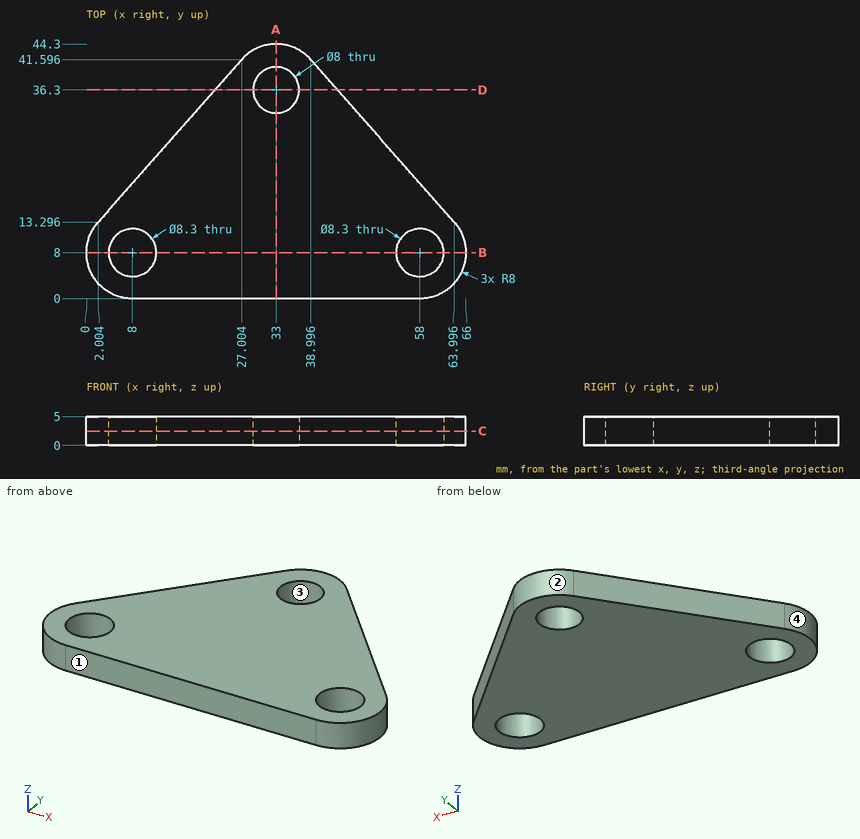
Check sheet for the drawn part. Datum: minimum x, y, z corner. Units: mm. Give positions to 0.01 mm unless a question says otherwise; leave off trailing zeros. Write each loop counter-clockwise with the first axis right and the second up, starting at its lowest first coordinate (ties: lowest second). Pieces come first, ordered by that corner, then holes. Notation, with made-up numbers: (26, 22.25) -> (69, 22.25) arc R7 cw to (69, 32.25) -> close; hole circle Ø11 at (9, 53.5). An arc over 180 degrees is marked (long way). Use one line per item in the form item = value. Start each with the question number.
1. Section check C-C (z = 2.5). Count the separate pieces of the cut face and the enclosed holes in it, and give its area (3 significant figures).
2. Go/stop test with flat-tipped pins: P1, Ø9, axis at x = 33, y = 36.3, coming from the +Z side; P2, Ø3, axis at y = 29.5, z = 4, coming from the -X side (1 decimal); P3, Ø3, axis at x = 7, z = 2.5, coming from the +Y side. Record where each tip stops, or that it passes through.
3. Section check A-A (x = 33). Record the cut outline in (y, z).
4. Thickness scan on line 1 along Y through (x, z) = (33, 2.9); line 2 along X through (y, z) = (7, 4.15); line 3 along X through (y, z) = (5.5, 2.35). Record the ranges inside material, lowest first. Write a range as from..to.
5. Section check B-B (y = 8). Record the cut outline in (x, z).
6. Mould release check, pull along X, two halves, no side actions. Record for the marked faces 1, 2, 3 and 4: pulls with the +X half, pulls with the -X half, needs draft (parallel to the pull), parting line crosses it, or undercut.
7. Section check D-D (y = 36.3). Record the cut outline in (x, z) (1 decimal).
Conclusion:
q1.separate_pieces = 1
q1.enclosed_holes = 3
q1.area = 1,750 mm²
q2.P1 = 5
q2.P2 = 15
q2.P3 = 20.65
q3.outline = (0, 0) -> (32.3, 0) -> (32.3, 5) -> (0, 5) -> close; (40.3, 0) -> (44.3, 0) -> (44.3, 5) -> (40.3, 5) -> close
q4.line_1 = 0..32.3, 40.3..44.3
q4.line_2 = 0.06..3.97, 12.03..53.97, 62.03..65.94
q4.line_3 = 0.4..4.69, 11.31..54.69, 61.31..65.6
q5.outline = (0, 0) -> (3.85, 0) -> (3.85, 5) -> (0, 5) -> close; (12.15, 0) -> (53.85, 0) -> (53.85, 5) -> (12.15, 5) -> close; (62.15, 0) -> (66, 0) -> (66, 5) -> (62.15, 5) -> close
q6.face_1 = needs draft
q6.face_2 = parting line crosses it
q6.face_3 = undercut
q6.face_4 = pulls with the -X half
q7.outline = (22.3, 0) -> (29, 0) -> (29, 5) -> (22.3, 5) -> close; (37, 0) -> (43.7, 0) -> (43.7, 5) -> (37, 5) -> close
